Verification items for this drawing (mm, ordinates from the low corner). A direction names the side the tool comes from. Give positions to 0.01 mm unless a question says otherwise; leave off trailing zeros. Order: outer loops, then holes, each group sorted by start corner. A loop starts at its lowest first (then second) coordinate and runs counter-clockwise, first axis right, second up.
(1) Mould release check, pull along Y, two halves, no side actions. Record for the marked faces 4, 5, 6 and 7: pulls with the +Y half, pulls with the -Y half, needs draft (parallel to the pull), parting line crosses it, or undercut.
(2) Gauge pin test, flat ends, axial feed: pin 1 (5 mm diameter, centred on x = 9, z = 9.5, fed in from -Y); pin 2 (6.5 mm diameter, centred on x = 27, y = 63, fed in from +Z); pin 3 (19 mm diameter, centred on x = 28.5, y = 62.5, fed in from +Z); pin 4 (4 mm diameter, centred on x = 25.5, z = 13, fed in from +Y). Record the tip position at first contact, or that the pin passes through.
(3) Scan lines: L1, parallel to Y at x = 27, z = 12.5; L2, parallel to Y at x = 27, z = 3.75; L3, parallel to Y at x = 24.5, z = 10.5. Record each from-to range of solid material in increasing order.
(4) Sectioned sample at D-D on z = 3. Record the cut outline in (x, y).
(5) Access from +Z, -Z, +X, -X, +Y, -Y to the whole of each face (thin tool, end or side, straight path). Record for the marked faces 1, 2 and 3.
(6) Sectioned sample at B-B on y = 61. Record the cut outline in (x, z).
(7) Sectioned sample at A-A on z = 9. Record the cut outline in (x, y).
(8) Sectioned sample at C-C on x = 27. Record the cut outline in (y, z), plus the area to 3 significant figures.
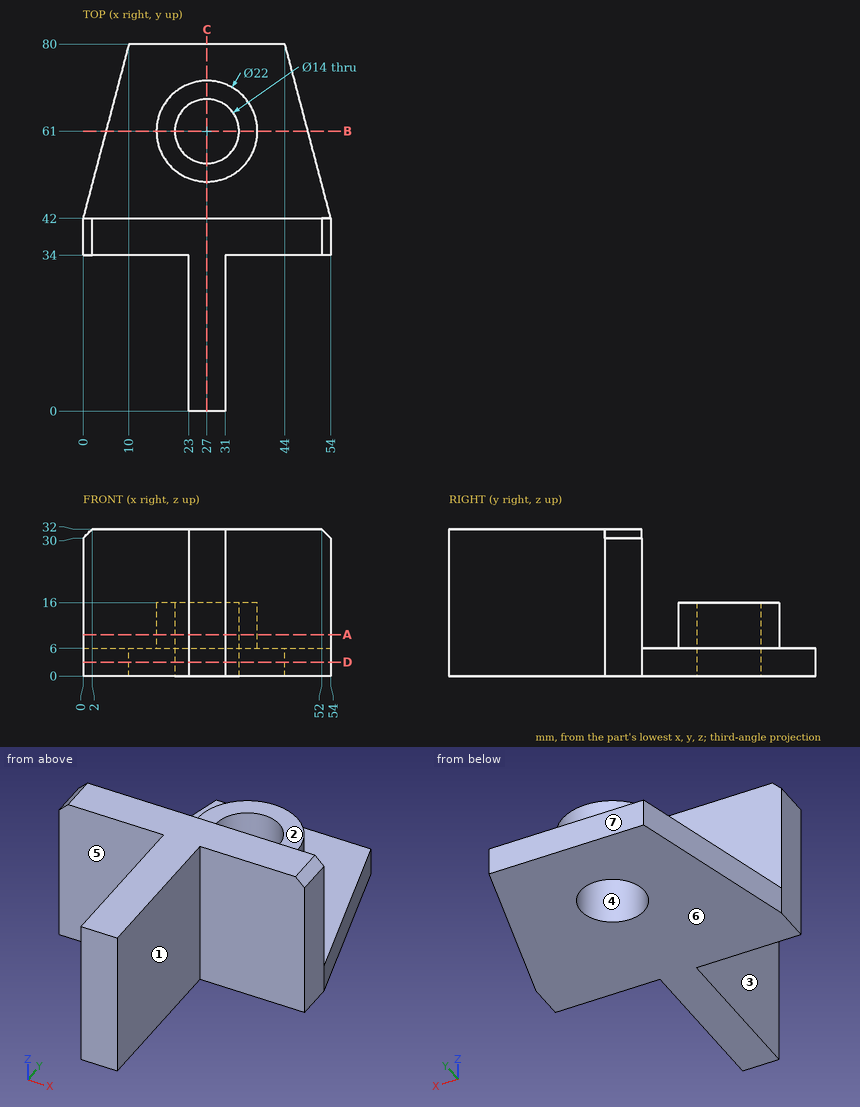
Ans:
1. face 4: undercut
1. face 5: pulls with the -Y half
1. face 6: needs draft
1. face 7: pulls with the +Y half
2. pin 1: stops at y = 34
2. pin 2: passes through
2. pin 3: stops at z = 16
2. pin 4: stops at y = 72
3. L1: y = 0 to 42, 50 to 54, 68 to 72
3. L2: y = 0 to 54, 68 to 80
3. L3: y = 0 to 42, 50.29 to 54.46, 67.54 to 71.71
4. outline: (0, 34) - (23, 34) - (23, 0) - (31, 0) - (31, 34) - (54, 34) - (54, 42) - (44, 80) - (10, 80) - (0, 42) - close; hole circle Ø14 at (27, 61)
5. face 1: +Z, -Z, +X, -Y
5. face 2: +Z, +X, -X, +Y
5. face 3: +Z, -Z, -X, -Y
6. outline: (5, 0) - (20, 0) - (20, 16) - (16, 16) - (16, 6) - (5, 6) - close; (34, 0) - (49, 0) - (49, 6) - (38, 6) - (38, 16) - (34, 16) - close
7. outline: (0, 34) - (23, 34) - (23, 0) - (31, 0) - (31, 34) - (54, 34) - (54, 42) - (0, 42) - close; circle Ø22 at (27, 61); hole circle Ø14 at (27, 61)
8. outline: (0, 0) - (54, 0) - (54, 16) - (50, 16) - (50, 6) - (42, 6) - (42, 32) - (0, 32) - close; (68, 0) - (80, 0) - (80, 6) - (72, 6) - (72, 16) - (68, 16) - close
8. area: 1,570 mm2
